Here's how the part is built. I have some questions about the finished solid (model axes, mm). Give positions to 0.01 mm unless a question says otherwise; leave off trailing zeros. Write each loop counter-clockwise with the first axis right and the second up, starting at its lowest first coordinate (ties: lowest second). Pieces come first, ordered by that corner, then holes. Notation, with made-up numbers: (-7, -17) - (28, -17) arc R32 cw to (28, 12) - close; hole circle Ø11 at (23, 1.5). An arc over 180 degrees is marked (long way). Write each question's results on one line, items separated by ' | '. Start each with the question number.
Item 1: We'd pull the mould along Y, two halves only. Please class faces 1 (the flat face through (0, 4, 1)), 2 (the flat face through (10, 0, 1)), 3 (the cylindrical face through (1.698, 4.582, 0.805)): +Y half, -Y half, draft (parallel to the pull), parting line (faces both ways), or undercut.
Item 2: Suppose I cut it at D-D on x = 17.78. List the corners of the cut face in (y, z) for me, then the cut area to 3 significant figures.
Item 3: Please list where these lines run through material, in increasing order: line 1 along Y through (x, z) = (10.16, 1.1); line 2 along X through (y, z) = (3, 0.9); line 3 along Y through (x, z) = (12.25, 0.8).
Item 4: Suppose I cut it at B-B on x = 7.62. List the corners of the cut face in (y, z) for me, then the cut area to 3 significant figures.
Item 5: Suppose I cut it at A-A on z = 0.6. List the corners of the cut face in (x, y) for me.
Item 6: Suppose I cut it at C-C on y = 4.75. List the corners of the cut face in (x, z) for me, then the cut area to 3 significant figures.
```python
from build123d import *

# Parameters (mm, degrees)
SKETCH1_W           = 20.32
SKETCH1_H           = 7.62
SKETCH1_R           = 0.508
BOSS_EXTRUDE1_DEPTH = 1.5875
SKETCH2_R           = 1.143
CUT_EXTRUDE1_DEPTH  = 22.759755427


with BuildPart() as part:
    # Sketch1 → Boss-Extrude1 (new body)
    with BuildSketch(Plane.XY):
        with Locations((10.16, 3.81)):
            Rectangle(SKETCH1_W, SKETCH1_H)
        with Locations((2.54, 3.81)):
            Circle(SKETCH1_R, mode=Mode.SUBTRACT)
        with Locations((5.08, 3.81)):
            Circle(SKETCH1_R, mode=Mode.SUBTRACT)
        with Locations((7.62, 3.81)):
            Circle(SKETCH1_R, mode=Mode.SUBTRACT)
        with Locations((10.16, 3.81)):
            Circle(SKETCH1_R, mode=Mode.SUBTRACT)
        with Locations((12.7, 3.81)):
            Circle(SKETCH1_R, mode=Mode.SUBTRACT)
        with Locations((15.24, 3.81)):
            Circle(SKETCH1_R, mode=Mode.SUBTRACT)
        with Locations((17.78, 3.81)):
            Circle(SKETCH1_R, mode=Mode.SUBTRACT)
    extrude(amount=BOSS_EXTRUDE1_DEPTH)

    # Sketch2 → Cut-Extrude1 (cut, through all)
    with BuildSketch(Plane.XY.offset(1.5875)):
        with Locations((2.54, 3.81)):
            Circle(SKETCH2_R)
        with Locations((17.78, 3.81)):
            Circle(SKETCH2_R)
    extrude(amount=-CUT_EXTRUDE1_DEPTH, mode=Mode.SUBTRACT)


solid = part.part
```
Checked values:
1) face 1: draft | face 2: -Y half | face 3: undercut
2) outline: (0, 0) - (2.67, 0) - (2.67, 1.59) - (0, 1.59) - close; (4.95, 0) - (7.62, 0) - (7.62, 1.59) - (4.95, 1.59) - close | area: 8.47 mm^2
3) line 1: y = 0 to 3.3, 4.32 to 7.62 | line 2: x = 0 to 1.73, 3.35 to 16.97, 18.59 to 20.32 | line 3: y = 0 to 3.57, 4.05 to 7.62
4) outline: (0, 0) - (3.3, 0) - (3.3, 1.59) - (0, 1.59) - close; (4.32, 0) - (7.62, 0) - (7.62, 1.59) - (4.32, 1.59) - close | area: 10.5 mm^2
5) outline: (0, 0) - (20.32, 0) - (20.32, 7.62) - (0, 7.62) - close; hole circle Ø2.29 at (2.54, 3.81); hole circle Ø1.02 at (5.08, 3.81); hole circle Ø1.02 at (7.62, 3.81); hole circle Ø1.02 at (10.16, 3.81); hole circle Ø1.02 at (12.7, 3.81); hole circle Ø1.02 at (15.24, 3.81); hole circle Ø2.29 at (17.78, 3.81)
6) outline: (0, 0) - (1.89, 0) - (1.89, 1.59) - (0, 1.59) - close; (3.19, 0) - (17.13, 0) - (17.13, 1.59) - (3.19, 1.59) - close; (18.43, 0) - (20.32, 0) - (20.32, 1.59) - (18.43, 1.59) - close | area: 28.1 mm^2
